Source: CAD feature listing. Evaluate the final solid. Frame: model axes, mm. A direction names the side the tool comes from. Round coordinates to 2 decimals unless told otherwise and drop trailing zeros. Order: outer loops, then holes, each group sorted by start corner. A loop starts at its lowest first (then second) coordinate and runs counter-clockwise, first axis right, second up. Notation, with made-up numbers: (-35, 44.25) - (-28, 44.25) arc R16 cw to (-28, 48.25) - close; hole circle Ø8 at (-29, 70.25). An arc over 180 degrees is marked (long way). Return JSON: item names as keys, results as strings. Group by question number.
1) Access query for faces 5 (the cylindrical face through (-94.994, -1.045, 0.507)), 6 (the flat face through (-105, -34, 1)), 7 (the cylindrical face through (-80.303, 71.367, 3.944)). Directions: +Z, -Z, +X, -X, +Y, -Y. A direction counts if a zero-diameter tool reaches every point of the face in a straight line with its end or side. Return the directions, or none.
2) Contact query for flat-ended pins moving along their axis: P1, Ø6, axis at x = -98, y = -31.5, coming from the +Z side; P2, Ø2.5, axis at x = -107, z = 1.5, coming from the -Y side; P3, Ø5, axis at x = -99, z = 13.5, coming from the +Y side; P4, Ø8, axis at x = -96.5, y = -30, coming from the -Z side. Output: stop coordinate, or through.
3) Ray query, line 1 (Y direction, x = -80, z = 5.75); line 2 (Y direction, x = -80, z = 5); line 3 (Y direction, x = -76.5, z = 3). Return the intervals inside material, ascending. Write a range as from..to.
4) Section A-A, the plane y = 0. Return loops of the section in (x, z) (3 decimals), plus the area to 3 significant figures.
5) Mould query, pull axis Y, two halves, no side actions, for faces 1 (the flat face through (-97, 1, 0)), 2 (the cylindrical face through (-96, -30, 1)), 3 (the flat face through (-77, -77, 7)), 4 (the cylindrical face through (-96, 30, 1)). Classes: pulls with the +Y half, pulls with the -Y half, needs draft (parallel to the pull), parting line crosses it, or undercut.
```python
from build123d import *

# Parameters (mm, degrees)
REVOLUTION_ANGLE = 90
POCKET_DEPTH     = 3
SKETCH002_R      = 1.4
POCKET001_DEPTH  = 8


with BuildPart() as part:
    # Sketch → Revolution (revolve, symmetric)
    with BuildSketch(Plane.XZ) as revolution_sk:
        with BuildLine():
            Line((-95, 0), (-115, 0))
            Line((-115, 0), (-115, 18))
            Line((-115, 18), (-112, 18))
            ThreePointArc((-112, 18), (-104.619043, 8.380957), (-95, 1))
            Line((-95, 0), (-95, 1))
        make_face()
    revolve(axis=Axis((0, 0, 0), (0, 0, 1)), revolution_arc=REVOLUTION_ANGLE / 2)
    revolve(revolution_sk.sketch, axis=Axis((0, 0, 0), (0, 0, -1)), revolution_arc=REVOLUTION_ANGLE / 2)

    # Sketch001 (on Face1 of Revolution) → Pocket (cut)
    with BuildSketch(Plane(origin=(0, 0, 0), x_dir=(1, 0, 0), z_dir=(0, 0, -1))):
        with BuildLine():
            ThreePointArc((-110, 34), (-114, 30), (-110, 26))
            Line((-110, 26), (-100, 26))
            ThreePointArc((-100, 26), (-96, 30), (-100, 34))
            Line((-110, 34), (-100, 34))
        make_face()
        with BuildLine():
            ThreePointArc((-110, -26), (-114, -30), (-110, -34))
            Line((-110, -34), (-100, -34))
            ThreePointArc((-100, -34), (-96, -30), (-100, -26))
            Line((-110, -26), (-100, -26))
        make_face()
    extrude(amount=-POCKET_DEPTH, mode=Mode.SUBTRACT)

    # Sketch002 (on Face1 of Pocket) → Pocket001 (cut)
    with BuildSketch(Plane(origin=(0, 0, 0), x_dir=(1, 0, 0), z_dir=(0, 0, -1))):
        with Locations((-80, 70)):
            Circle(SKETCH002_R)
        with Locations((-80, -70)):
            Circle(SKETCH002_R)
        with Locations((-110, 0)):
            Circle(SKETCH002_R)
        with Locations((-100, -40)):
            Circle(SKETCH002_R)
        with Locations((-100, 40)):
            Circle(SKETCH002_R)
    extrude(amount=-POCKET001_DEPTH, mode=Mode.SUBTRACT)


solid = part.part
```
Geometry check:
{
 "1": {"face 5": "+Z, -Z, +X", "face 6": "-Z, -X", "face 7": "-Z"},
 "2": {"P1": "z = 9.76", "P2": "y = -45.19", "P3": "y = 62.55", "P4": "z = 0"},
 "3": {"line 1": "-80..-71.4, -68.6..-62.89, 62.89..68.6, 71.4..80", "line 2": "-80..-71.4, -68.6..-61.4, 61.4..68.6, 71.4..80", "line 3": "-76.5..-61.51, 61.51..76.5"},
 "4": {"outline": "(-115, 0) - (-111.4, 0) - (-111.4, 8) - (-108.6, 8) - (-108.6, 0) - (-95, 0) - (-95, 1) arc R46.445 cw to (-112, 18) - (-115, 18) - close", "area": "168 mm2"},
 "5": {"face 1": "needs draft", "face 2": "undercut", "face 3": "pulls with the -Y half", "face 4": "undercut"}
}
